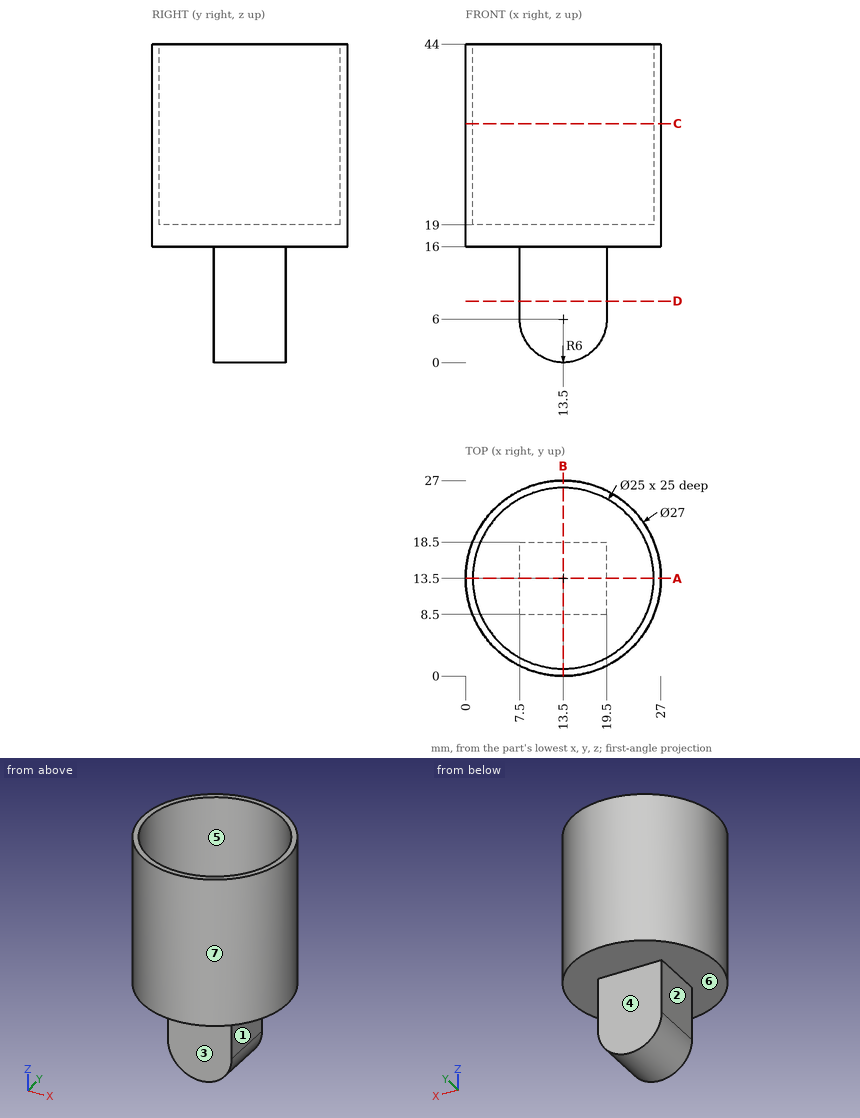
Here's the drawing with two shaded views (mm, measured from the low corner). I have some questions. A direction names the side the tool comes from. Give positions to 0.01 mm unless a question says otherwise; leave off trailing zeros. Loops run counter-clockwise (first coordinate to the right, second up) from the corner with the lowest first, then second, coordinate; pieces in that order, holes last. Notation, with made-up numbers: (0, -16) - (11, -16) arc R11 ccw to (11, -9) - close; hole circle Ø5 at (-0.75, 55.5). An arc over 180 degrees is marked (long way). Answer in a Markdown table with one row per item. Add a question column.
Q1. If we section it at A-A (y = 13.5): List the corners of the cut face in (x, z) for me, plus the area to 3 significant figures.
Q2. Which directions (+Z, -Z, +X, -X, +Y, -Y) give clear straight access to the entire face, cutting with the end or side of a thin tool? Please do the marked faces 1, 2, 3 and 4.
Q3. If we section it at C-C (z = 33): List the corners of the cut face in (x, y) for me, plus the area to 3 significant figures.
Q4. If we section it at B-B (x = 13.5): List the corners of the cut face in (y, z) for me.
Q5. We'd pull the mould along Y, two halves only. Please class the marked faces 5, 6 and 7: +Y half, -Y half, draft (parallel to the pull), parting line (faces both ways), or undercut.
Q6. Please list where these lines run through material, in increasing order: L1, parallel to Y at x = 13.5, z = 33.5; L2, parallel to Z at x = 4.5, y = 17.25; L3, parallel to Y at x = 2, z = 27.5. Write a range as from..to.
Q7. If we section it at D-D (z = 8.5): List the corners of the cut face in (x, y) for me.
Q8. For pin 1 (3 mm diameter, centred on x = 7.5, y = 14.5, fed in from +Z); pin 2 (2 mm diameter, centred on x = 10, z = 11, fed in from +Y); pin 3 (1 mm diameter, centred on x = 9, z = 27.5, fed in from +Y); pin 4 (1.5 mm diameter, centred on x = 22, z = 13.5, fed in from +Y), each with a flat end and sliding along its axis, tell me the tip position at first contact or that it passes through.
The answers:
| question | item | result |
|---|---|---|
| 1 | outline | (0, 16) - (7.5, 16) - (7.5, 6) arc R6 ccw to (19.5, 6) - (19.5, 16) - (27, 16) - (27, 44) - (26, 44) - (26, 19) - (1, 19) - (1, 44) - (0, 44) - close |
| 1 | area | 308 mm^2 |
| 2 | face 1 | -Z, +X, +Y, -Y |
| 2 | face 2 | -Z, -X, +Y, -Y |
| 2 | face 3 | -Z, +X, -X, -Y |
| 2 | face 4 | -Z, +X, -X, +Y |
| 3 | outline | circle Ø27 at (13.5, 13.5); hole circle Ø25 at (13.5, 13.5) |
| 3 | area | 81.7 mm^2 |
| 4 | outline | (0, 16) - (8.5, 16) - (8.5, 0) - (18.5, 0) - (18.5, 16) - (27, 16) - (27, 44) - (26, 44) - (26, 19) - (1, 19) - (1, 44) - (0, 44) - close |
| 5 | face 5 | undercut |
| 5 | face 6 | draft |
| 5 | face 7 | parting line |
| 6 | L1 | y = 0..1, 26..27 |
| 6 | L2 | z = 16..19 |
| 6 | L3 | y = 6.43..8.6, 18.4..20.57 |
| 7 | outline | (7.5, 8.5) - (19.5, 8.5) - (19.5, 18.5) - (7.5, 18.5) - close |
| 8 | pin 1 | stops at z = 19 |
| 8 | pin 2 | stops at y = 18.5 |
| 8 | pin 3 | stops at y = 26.39 |
| 8 | pin 4 | passes through |
